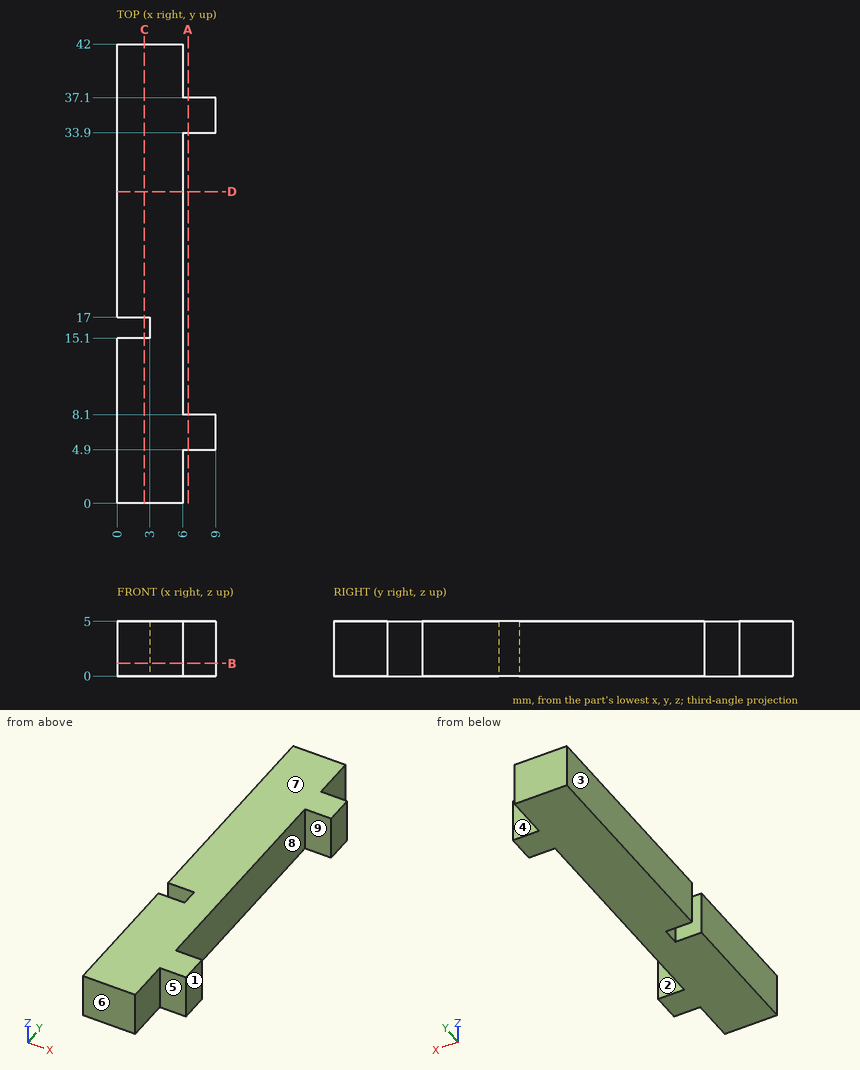
The figure shows three views and two pictorial views of one solid part (mm, origin at its lowest corner). Answer the questions. A direction names the side the tool comes from. Give positions to 0.01 mm unless a question says otherwise; leave off trailing zeros. Write each loop counter-clockwise with the first axis right and the second up, starting at its lowest first coordinate (ties: lowest second). Pieces come first, ordered by that corner, then holes. Notation, with made-up numbers: (-13, 56.25) -> (6, 56.25) arc R20 cw to (6, 78.25) -> close; hole circle Ø7 at (7, -33). An arc over 180 degrees is marked (long way). Answer as a JSON object with one key per item and string values.
1) Flat-ended cylindrical pins translate along their axes: pin 1 Ø2.5 at (x, z) = (8, 2) entering from +Y; pin 2 Ø1.5 at (x, z) = (7.5, 1.5) entering from -Y; pin 3 Ø1 at (y, z) = (16, 1.5) entering from -X. Find the tip coordinate at first contact, or state that the pin passes through.
Findings below:
{"pin 1": "stops at y = 37.1", "pin 2": "stops at y = 4.9", "pin 3": "stops at x = 3"}
2) A tool of negligible diameter and unlimited length cuts with its end or side. For the marked faces 1, 2, 3, 4 and 5, from which of +Z, -Z, +X, -X, +Y, -Y can it reach the whole face along a straight path? Write none if from no direction.
Findings below:
{"face 1": "+Z, -Z, +X, +Y, -Y", "face 2": "+Z, -Z, +X", "face 3": "+Z, -Z, -X, +Y, -Y", "face 4": "+Z, -Z, +X, +Y", "face 5": "+Z, -Z, +X, -Y"}
3) Straight lines are drawn through the part: probe 1 along Y at (x, z) = (1.5, 3.7); probe 2 along X at (y, z) = (19.5, 1.35). For each, find the intervals that lie inside material, in ascending order. Write a range as from..to.
Findings below:
{"probe 1": "y = 0..15.1, 17..42", "probe 2": "x = 0..6"}
4) Section C-C on x = 2.5 is taken. Write down the section's boundary in (y, z), then the cut area to 4 significant figures.
Findings below:
{"outline": "(0, 0) -> (15.1, 0) -> (15.1, 5) -> (0, 5) -> close; (17, 0) -> (42, 0) -> (42, 5) -> (17, 5) -> close", "area": "200.5 mm^2"}
5) Section B-B on z = 1.15 is taken. Write down the section's boundary in (x, y), then the cut area to 4 significant figures.
Findings below:
{"outline": "(0, 0) -> (6, 0) -> (6, 4.9) -> (9, 4.9) -> (9, 8.1) -> (6, 8.1) -> (6, 33.9) -> (9, 33.9) -> (9, 37.1) -> (6, 37.1) -> (6, 42) -> (0, 42) -> (0, 17) -> (3, 17) -> (3, 15.1) -> (0, 15.1) -> close", "area": "265.5 mm^2"}
6) For a pull along Y with two mould halves and no side action, classify the marked faces 6, 7, 8 and 9 as pulls with the +Y half, pulls with the -Y half, needs draft (parallel to the pull), parting line crosses it, or undercut.
Findings below:
{"face 6": "pulls with the -Y half", "face 7": "needs draft", "face 8": "undercut", "face 9": "undercut"}
7) Section D-D on y = 28.5 is taken. Write down the section's boundary in (x, z), then the cut area to 3 significant figures.
Findings below:
{"outline": "(0, 0) -> (6, 0) -> (6, 5) -> (0, 5) -> close", "area": "30.0 mm^2"}
8) Section A-A on x = 6.5 is taken. Write down the section's boundary in (y, z), then the cut area to 3 significant figures.
Findings below:
{"outline": "(4.9, 0) -> (8.1, 0) -> (8.1, 5) -> (4.9, 5) -> close; (33.9, 0) -> (37.1, 0) -> (37.1, 5) -> (33.9, 5) -> close", "area": "32.0 mm^2"}
